Input: part model. Units: mm. Frame: model coordinates. Face numbers are marked on the shaded views. Coordinates: 2 decimals unless noted, no trailing zeros. Order: outer loops, then holes, each group sorted by start corner. A loop starts at its lowest first (then second) coordinate and runs counter-clockwise, first axis right, second up. Notation, with made-up numbers: (-35, 81) -> (20, 81) arc R16 cw to (20, 100) -> close; hole circle Ø6 at (-21, -36.75). An arc over 180 degrees is marked (long way). Use one line per item in the form item = value. Start each with the question number.
1) Section query A-A on x = 0. Output: boundary loops of the cut face in (y, z), then the cut area to 3 significant figures.
2) Section query C-C on x = -7. Output: boundary loops of the cut face in (y, z), then the cut area to 3 significant figures.
3) Section query D-D on z = -13. Output: boundary loops of the cut face in (x, y), then the cut area to 3 significant figures.
4) Draft query along X for the marked faces 1, 2 and 3. Return one class per face: pulls with the +X half, pulls with the -X half, needs draft (parallel to the pull), parting line crosses it, or undercut.
5) Section query B-B on z = 0. Output: boundary loops of the cut face in (x, y), then the cut area to 3 significant figures.
6) Pin query (flat end, axial travel): pin 1 (10 mm diameter, centred on x = 2, z = 7, fed in from -Y); pin 2 (3 mm diameter, centred on x = -8.5, y = -3, fed in from +Z); pin 3 (2 mm diameter, centred on y = -2.5, z = 3.5, fed in from +X). Return the tip coordinate at first contact, or that it passes through.
7) Ray query, line 1 along Y through (x, z) = (0, -14.65); line 2 along X through (y, z) = (-2.2, -14); line 3 along X through (y, z) = (-2, 3.5). Return the intervals inside material, ascending.
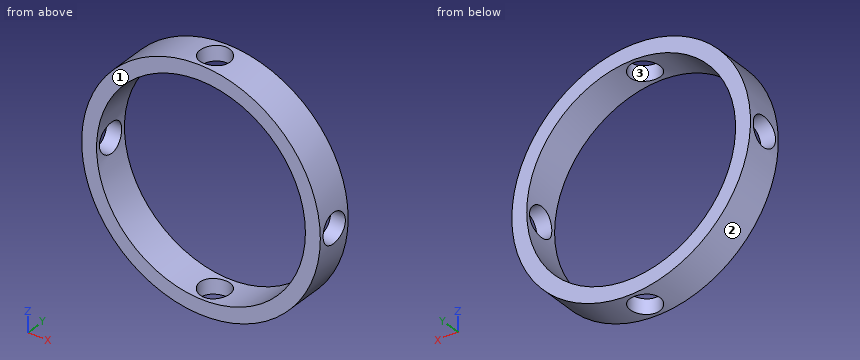
from build123d import *

# Parameters (mm, degrees)
F0_R     = 16
F0_R_2   = 14
F1_DEPTH = 5
F4_D     = 4
F7_D     = 4


with BuildPart() as f1:
    # F0 (on Front) → F1 (new body)
    with BuildSketch(Plane.XZ):
        Circle(F0_R)
        Circle(F0_R_2, mode=Mode.SUBTRACT)
    extrude(amount=F1_DEPTH)

    # F4 (through all)
    with Locations(Plane.YZ.offset(16)):
        with Locations((-2.5, 0)):
            Hole(F4_D / 2)

    # F7 (through all)
    with Locations(Plane.XY.offset(16)):
        with Locations((0, -2.5)):
            Hole(F7_D / 2)


solid = f1.part
Answers below:
q1.outline = (-5, -16) -> (-4.5, -16) -> (-4.5, -14) -> (-5, -14) -> close; (-5, 14) -> (-4.5, 14) -> (-4.5, 16) -> (-5, 16) -> close; (-0.5, -16) -> (0, -16) -> (0, -14) -> (-0.5, -14) -> close; (-0.5, 14) -> (0, 14) -> (0, 16) -> (-0.5, 16) -> close
q1.area = 4.00 mm^2
q2.outline = (-5, -14.39) -> (0, -14.39) -> (0, -12.12) -> (-5, -12.12) -> close; (-5, 12.12) -> (0, 12.12) -> (0, 14.39) -> (-5, 14.39) -> close
q2.area = 22.6 mm^2
q3.outline = (-9.33, -5) -> (-5.2, -5) -> (-5.2, 0) -> (-9.33, 0) -> close; (5.2, -5) -> (9.33, -5) -> (9.33, 0) -> (5.2, 0) -> close
q3.area = 41.3 mm^2
q4.face_1 = needs draft
q4.face_2 = parting line crosses it
q4.face_3 = undercut
q5.outline = (-16, -5) -> (-14, -5) -> (-14, -4.5) -> (-16, -4.5) -> close; (-16, -0.5) -> (-14, -0.5) -> (-14, 0) -> (-16, 0) -> close; (14, -5) -> (16, -5) -> (16, -4.5) -> (14, -4.5) -> close; (14, -0.5) -> (16, -0.5) -> (16, 0) -> (14, 0) -> close
q5.area = 4.00 mm^2
q6.pin_1 = through
q6.pin_2 = 14.39
q6.pin_3 = 15.8
q7.line_1 = -5 to -4.5, -0.5 to 0
q7.line_2 = -7.75 to -1.98, 1.98 to 7.75
q7.line_3 = -15.61 to -13.56, 13.56 to 15.61
